Answer from the drawing. Dimensions are ordinates in mm from the lowest x, y and z of the part. Round coordinates to 2 decimals unless told otherwise and drop trailing zeros. Write each loop counter-clockwise with the first axis right and the second up, starting at its lowest first coordinate (ties: lowest second). Pieces come first, ordered by that corner, then holes. Notation, with made-up numbers: (57.25, 72.5) -> (79.25, 72.5) arc R5 cw to (79.25, 77.5) -> close; hole circle Ø8 at (55.25, -30.75). An arc over 180 degrees is marked (long way). Return JSON: item names as keys, results as strings. Group by question number.
(1) The mould has two halves that part along X. Classify the marked faces 1, 2 and 3: released by +X, released by -X, zero draft, split by the parting line, or undercut.
(2) A cutting plane is placed at D-D on x = 39. Give the vertices of the cut face in (y, z), then the cut area to 3 significant figures.
(3) Straight lines are drawn through the part: line 1 (X direction, y = 3.25, z = 4); line 2 (X direction, y = 8.5, z = 11) (1 decimal); line 3 (Y direction, x = 28.5, z = 23). For each, find the intervals that lie inside material, in ascending order.
(4) A cutting plane is placed at C-C on y = 5.75. Give the vertices of the cut face in (x, z), then the cut area to 3 significant figures.
(5) A cutting plane is placed at A-A on y = 3. Give the vertices of the cut face in (x, z), then the cut area to 3 significant figures.
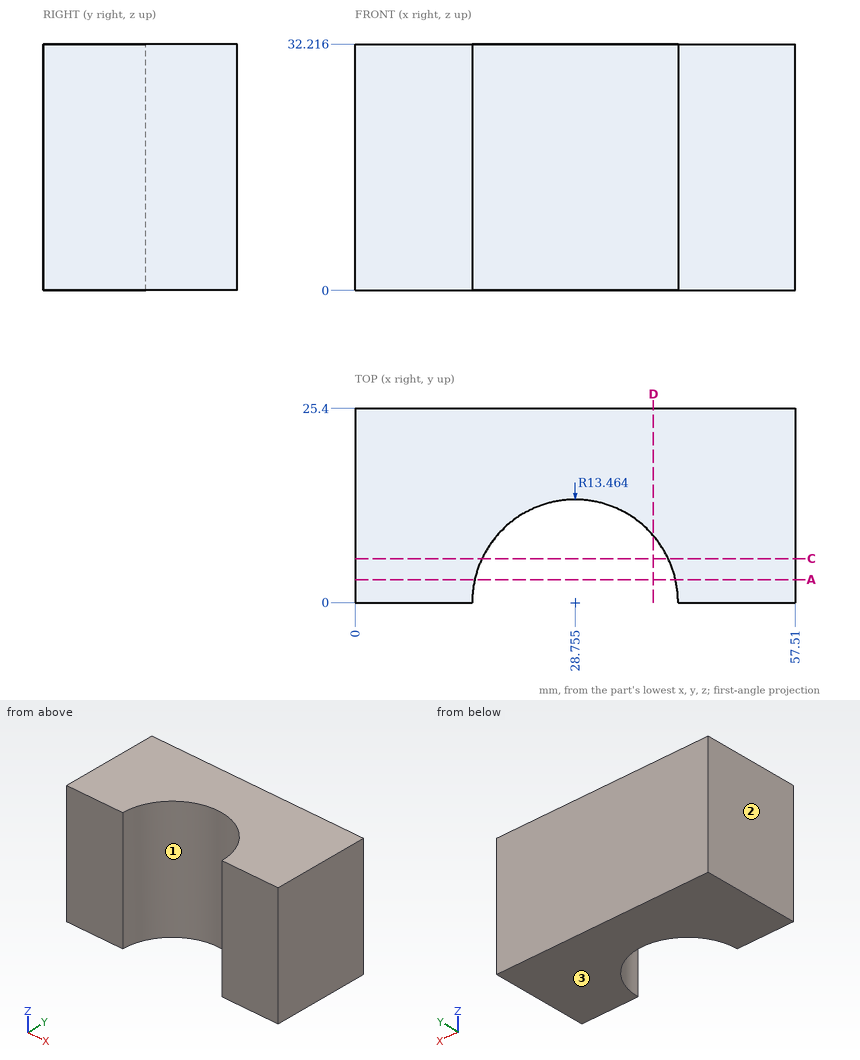
Checks:
{
 "1": {"face 1": "undercut", "face 2": "released by -X", "face 3": "zero draft"},
 "2": {"outline": "(8.74, 0) -> (25.4, 0) -> (25.4, 32.22) -> (8.74, 32.22) -> close", "area": "537 mm^2"},
 "3": {"line 1": "x = 0 to 15.69, 41.82 to 57.51", "line 2": "x = 0 to 18.3, 39.2 to 57.5", "line 3": "y = 13.46 to 25.4"},
 "4": {"outline": "(0, 0) -> (16.58, 0) -> (16.58, 32.22) -> (0, 32.22) -> close; (40.93, 0) -> (57.51, 0) -> (57.51, 32.22) -> (40.93, 32.22) -> close", "area": "1,070 mm^2"},
 "5": {"outline": "(0, 0) -> (15.63, 0) -> (15.63, 32.22) -> (0, 32.22) -> close; (41.88, 0) -> (57.51, 0) -> (57.51, 32.22) -> (41.88, 32.22) -> close", "area": "1,010 mm^2"}
}
